Can you work these out from the model? Positions are in its coordinate system, mm. A direction names the side the tool comes from. Round coordinates to 2 decimals unless told otherwise and drop trailing zeros. Order: outer loops, then holes, each group sorted by start corner. A loop starts at its lowest first (then second) coordinate and runs counter-clockwise, first axis right, second up. Notation, with made-up numbers: M -7,30.25 L 33,30.25 A21 ccw 33,43.25 Z; hole C 6.25,64.25 d7. An arc over 180 degrees is marked long. One line per question, with ' | ' between items.
```python
from build123d import *

# Parameters (mm, degrees)
EXTRUDE_F_DEPTH    = 80
SKETCH2_R          = 1.75
CUT_EXTRUDE1_DEPTH = 6.1
CUT_EXTRUDE2_START = -6.1
SKETCH3_R          = 1.75
CUT_EXTRUDE2_DEPTH = 6.1


with BuildPart() as part:
    # Sketch1 → Extrude f (new body)
    with BuildSketch(Plane.XY):
        Polygon((4.041451884, 0), (2.020725942, 3.5), (-2.020725942, 3.5), (-4.041451884, 0), (-2.020725942, -3.5), (2.020725942, -3.5), align=None)
    extrude(amount=EXTRUDE_F_DEPTH)

    # Sketch2 → Cut-Extrude1 (cut)
    with BuildSketch(Plane.XY.offset(80)):
        Circle(SKETCH2_R)
    extrude(amount=-CUT_EXTRUDE1_DEPTH, mode=Mode.SUBTRACT)

    # Sketch3 → Cut-Extrude2 (cut)
    with BuildSketch(Plane(origin=(0, 0, 0), x_dir=(-1, 0, 0), z_dir=(0, 0, -1)).offset(CUT_EXTRUDE2_START)):
        with Locations(Location((0, 0, 0), (0, 0, 180))):
            Circle(SKETCH3_R)
    extrude(amount=CUT_EXTRUDE2_DEPTH, mode=Mode.SUBTRACT)


solid = part.part
```
(1) If we section it at B-B on y = 1: Please give me the cut outline in (x, z).
Final values:
outline: M -3.46,0 L -1.44,0 L -1.44,6.1 L 1.44,6.1 L 1.44,0 L 3.46,0 L 3.46,80 L 1.44,80 L 1.44,73.9 L -1.44,73.9 L -1.44,80 L -3.46,80 Z
(2) Will these pins go through, and if not, where does the flat tip stop? pin 1 Ø1.8 at (x, y) = (0, 0.5) entering from +Z; pin 2 Ø3 at (x, y) = (0, 0) entering from -Z; pin 3 Ø3 at (y, z) = (-2.5, 46.5) entering from +X.
Final values:
pin 1: z = 73.9 | pin 2: z = 6.1 | pin 3: x = 3.46
(3) If we section it at C-C on z = 46: Please give me the cut outline in (x, y), plus the area to 3 significant figures.
Final values:
outline: M -4.04,0 L -2.02,-3.5 L 2.02,-3.5 L 4.04,0 L 2.02,3.5 L -2.02,3.5 Z | area: 42.4 mm^2
(4) On a 3-axis mill with a long thin cutter (end or side, diameter ignored), from which of +Z, -Z, +X, -X, +Y, -Y can I reach the whole of each face in a straight line? I mean faces 1 (the flat face through (0, 0, 73.9)), 2 (the flat face through (1, 2, 0)). Say none if no direction works.
Final values:
face 1: +Z | face 2: -Z, +X, -X, +Y, -Y
(5) If we section it at A-A on x = 0: Please give me the cut outline in (y, z).
Final values:
outline: M -3.5,0 L -1.75,0 L -1.75,6.1 L 1.75,6.1 L 1.75,0 L 3.5,0 L 3.5,80 L 1.75,80 L 1.75,73.9 L -1.75,73.9 L -1.75,80 L -3.5,80 Z
(6) Thinking about a two-plate mould opening in X: for faces 3 (the flat face through (-3.045, -1.726, 39.44)), 4 (the flat face through (3, -1.8, 39.4)), 5 (the cylindrical face through (1.617, 0.67, 3.093)), 6 (the flat face through (0, 0, 6.1)), which applies, released by +X, released by -X, zero draft, split by the parting line, or undercut?
Final values:
face 3: released by -X | face 4: released by +X | face 5: undercut | face 6: undercut
(7) If we section it at D-D on x = 3: Please give me the cut outline in (y, z), plus the area to 3 significant figures.
Final values:
outline: M -1.8,0 L 1.8,0 L 1.8,80 L -1.8,80 Z | area: 289 mm^2
(8) Please list where these lines run through material, in increasing order: probe 1 along Y at (x, z) = (0, 2.5); probe 2 along X at (y, z) = (-1.25, 6); probe 3 along X at (y, z) = (-1, 57.5). Write a range as [from, to].
Final values:
probe 1: [-3.5, -1.75], [1.75, 3.5] | probe 2: [-3.32, -1.22], [1.22, 3.32] | probe 3: [-3.46, 3.46]
